Autodesk Inventor part; units mm, degrees
ref_plane "YZ Plane" through (0, 0, 0) normal (1, 0, 0) x (0, 1, 0)
ref_plane "XZ Plane" through (0, 0, 0) normal (0, 1, 0) x (-1, 0, 0)
ref_plane "XY Plane" through (0, 0, 0) normal (0, 0, 1) x (1, 0, 0)
sketch "Sketch1" plane through (0, 0, 0) normal (0, 1, 0) x (-1, 0, 0)
  line L0 (41.1895, 30.2734) -> (43.9395, 25.5103)
  line L1 (43.9395, 25.5103) -> (47.5768, 27.6103)
  line L2 (42.0768, 37.1366) -> (38.4395, 35.0366)
  line L3 (38.4395, 35.0366) -> (41.1895, 30.2734)
  arc A0 (46.0996, 30.1689) -> (43.5541, 34.578) centre (44.0588, 31.93) ccw
  line L4 (42.0768, 37.1366) -> (43.5541, 34.578)
  line L5 (46.0996, 30.1689) -> (47.5768, 27.6103)
  line L6 (40.2582, 36.0866) -> (43.5582, 36.0866) construction
  circle A1 centre (38.6082, 38.9445) radius 1.4
  line L7 (41.7517, 43.2997) -> (35.9493, 39.9497)
  line L8 (35.9493, 39.9497) -> (35.2173, 37.2177)
  line L9 (39.7286, 29.43) -> (35.2173, 37.2177)
  line L10 (44.4838, 42.5677) -> (41.7517, 43.2997)
  line L11 (44.9838, 41.7016) -> (44.4838, 42.5677)
  line L12 (44.9838, 41.7016) -> (48.976, 34.7869)
  circle A2 centre (47.4248, 23.7248) radius 1.4
  line L13 (52.7668, 24.2851) -> (46.9742, 20.9182)
  line L14 (46.9742, 20.9182) -> (44.24, 21.6423)
  line L15 (39.7286, 29.43) -> (44.24, 21.6423)
  line L16 (53.4908, 27.0193) -> (52.7668, 24.2851)
  line L17 (52.9883, 27.8839) -> (53.4908, 27.0193)
  line L18 (52.9883, 27.8839) -> (48.976, 34.7869)
  point P0 (34.2173, 38.9497)
  point P1 (43.4838, 44.2997)
  point P2 (45.245, 19.9132)
  point P3 (54.4959, 25.2902)
  dimension "d0" = 5
  dimension "d29" = 2.8
  dimension "d32" = 2
  dimension "d33" = 2
  dimension "d34" = 2
  dimension "d35" = 2
  dimension "d41" = 2.8
extrude "Extrusion1" add sketch "Sketch1" along normal blind 12
sketch "Sketch3" plane through (-38.4395, 2, 35.0366) normal (-0.8660254, 0, 0.5) x (0.5, 0, 0.8660254)
  line L0 (-11, 0) -> (0, 0)
  line L1 (-5.5, 0) -> (-5.5, 3.3)
  circle A0 centre (-5.5, 3.3) radius 1.65
  point P0 (-11.1228, -2)
  dimension "d20" = 3.3
  dimension "d21" = 3.3
extrude "Extrusion3" cut sketch "Sketch3" along normal through all
sketch "Sketch4" plane through (0, 0, 0) normal (0, -1, 0) x (1, 0, 0)
  line L0 (-42.0768, 37.1366) -> (-38.4395, 35.0366)
  line L1 (-38.4395, 35.0366) -> (-43.9395, 25.5103)
  line L2 (-43.9395, 25.5103) -> (-47.5768, 27.6103)
  line L3 (-47.5768, 27.6103) -> (-46.0996, 30.1689)
  arc A0 (-43.5541, 34.578) -> (-46.0996, 30.1689) centre (-44.0588, 31.93) ccw
  line L4 (-43.5541, 34.578) -> (-42.0768, 37.1366)
  circle A1 centre (-47.4248, 23.7248) radius 1.4
  circle A2 centre (-38.6082, 38.9445) radius 1.4
  line L5 (-44.24, 21.6423) -> (-35.2173, 37.2177)
  line L6 (-35.2173, 37.2177) -> (-35.9493, 39.9497)
  line L7 (-35.9493, 39.9497) -> (-41.7517, 43.2997)
  line L8 (-41.7517, 43.2997) -> (-44.4838, 42.5677)
  line L9 (-44.4838, 42.5677) -> (-48.976, 34.7869)
  line L10 (-48.976, 34.7869) -> (-53.4908, 27.0193)
  line L11 (-53.4908, 27.0193) -> (-52.7668, 24.2851)
  line L12 (-52.7668, 24.2851) -> (-46.9742, 20.9182)
  line L13 (-46.9742, 20.9182) -> (-44.24, 21.6423)
  point P0 (0, 0)
extrude "Extrusion4" add sketch "Sketch4" against normal blind 2 contours L0 L1 L2 L3 A0 L4 | A1 | A2
chamfer "Chamfer2" distance 2 angle 45 9 edges at (-53.1288, 0, 25.6522) (-51.2334, 0, 30.9031) (-46.7299, 0, 38.6773) (-43.1177, 0, 42.9337) (-38.8505, 0, 41.6247) (-35.5833, 0, 38.5837) (-39.7286, 0, 29.43) (-45.6071, 0, 21.2803) (-49.8705, 0, 22.6017)
properties part number "TSOP Holder Straight" material "ABS Plastic"
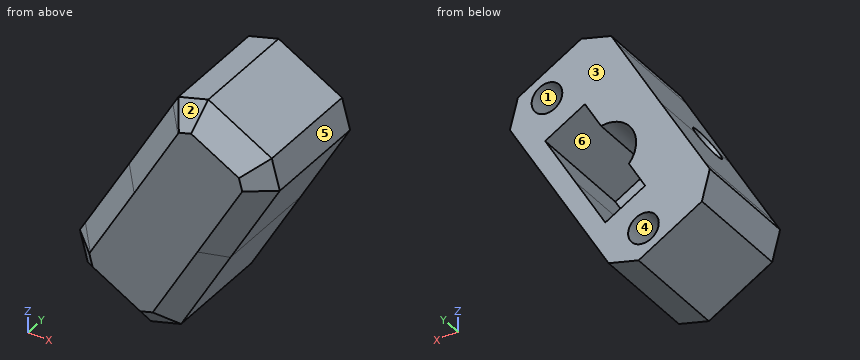
The listing builds one solid part. Answer for the finished solid, in the listing's coordinates (mm). Face numbers are marked on the shaded views. A direction names the side the tool comes from. Give positions to 0.01 mm unless a question says otherwise; leave off trailing zeros. Order: outer loops, then holes, each group sorted by start corner. A loop starts at its lowest first (then second) coordinate and runs counter-clockwise, first axis right, second up. Notation, with made-up numbers: (-18, -18.75) - (11, -18.75) arc R30 cw to (11, 8.25) - close; hole circle Ø10 at (-9, -6). An arc over 180 degrees is marked (long way). One line per item, written item: value. Start each with the question number.
1) A tool of negligible diameter and unlimited length cuts with its end or side. For the marked faces 5 and 6, from which of +Z, -Z, +X, -X, +Y, -Y can it reach the whole face along a straight path? Write none if from no direction.
2) A cutting plane is placed at A-A on y = 8.25. Give the vertices of the cut face in (x, z), then the cut area to 3 significant figures.
3) A cutting plane is placed at C-C on z = 29. Give the vertices of the cut face in (x, y).
4) A cutting plane is placed at D-D on x = -52. Give the vertices of the cut face in (y, z), then the cut area to 3 significant figures.
5) A cutting plane is placed at B-B on x = -38. Give the vertices of the cut face in (y, z), then the cut area to 3 significant figures.
6) The mould has two halves that part along Z. Classify the marked faces 1, 2, 3 and 4: released by +Z, released by -Z, zero draft, split by the parting line, or undercut.
7) Find the intervals of material crossed by L1, parallel to Z at x = -39, y = 9; L2, parallel to Z at x = -46.5, y = 4.5; L3, parallel to X at y = 10.5, z = 25, in increasing order.
8) Given pin 1 Ø1.4 at (x, z) = (-39, 38.5) entering from +Y; pin 2 Ø5 at (y, z) = (7, 23) entering from +X; pin 3 Ø2 at (x, y) = (-40, 3.5) entering from +Z, each flat-ended and moving along its own axis, determine where each tip first touches the part or whether it passes through.
Answer sheet:
1. face 5: +Z, +X, +Y, -Y
1. face 6: +Y
2. outline: (-53.49, 27.02) - (-52.77, 24.29) - (-46.97, 20.92) - (-44.24, 21.64) - (-39.73, 29.43) - (-35.22, 37.22) - (-35.95, 39.95) - (-41.75, 43.3) - (-44.48, 42.57) - (-44.98, 41.7) - (-48.98, 34.79) - (-52.99, 27.88) - close; hole circle Ø2.8 at (-47.42, 23.72); hole (-47.58, 27.61) - (-43.94, 25.51) - (-41.19, 30.27) - (-38.44, 35.04) - (-42.08, 37.14) - (-43.55, 34.58) arc R2.7 ccw to (-46.1, 30.17) - close; hole circle Ø2.8 at (-38.61, 38.94)
2. area: 162 mm2
3. outline: (-52.34, 2) - (-50.03, 0) - (-42.29, 0) - (-39.98, 2) - (-39.98, 12) - (-41.92, 12) - (-41.92, 2) - (-46.77, 2) - (-46.77, 12) - (-52.34, 12) - close
4. outline: (0.61, 26.82) - (1.11, 24.87) - (2, 23.84) - (12, 23.84) - (12, 29.58) - (2, 29.58) - (0.86, 27.31) - close
4. area: 62.1 mm2
5. outline: (0, 36.4) - (2, 32.41) - (12, 32.41) - (12, 37.68) - (2, 37.68) - (2, 40.21) - (12, 40.21) - (12, 41.13) - (2, 41.13) - (0, 38.82) - close
5. area: 73.1 mm2
6. face 1: undercut
6. face 2: released by +Z
6. face 3: zero draft
6. face 4: undercut
7. L1: z = 30.69 to 34.07, 35.36 to 37.6, 40.29 to 41.71
7. L2: z = 21.04 to 22.67, 24.78 to 26.99, 29.48 to 30.79, 35.01 to 39.08
7. L3: x = -52.96 to -48, -46.85 to -42.29
8. pin 1: stops at y = 2
8. pin 2: stops at x = -42.01
8. pin 3: stops at z = 42.87
